Job drawing, mm, ordinate dimensions from the low corner. One solid piece. Give positions to 0.01 mm unless a question says otherwise; leave off trailing zeros. Order: outer loops, then holes, each group sorted by start corner. A loop starts at its lowest first (then second) coordinate and runs counter-clockwise, first axis right, second up. Notation, with made-up numbers: (6.5, 26.25) - (47.5, 26.25) arc R9 cw to (47.5, 31.25) - close; hole circle Ø10 at (70.5, 16.25). An arc over 180 degrees is marked (long way). Use a Markdown table: item, result. Add a question column.
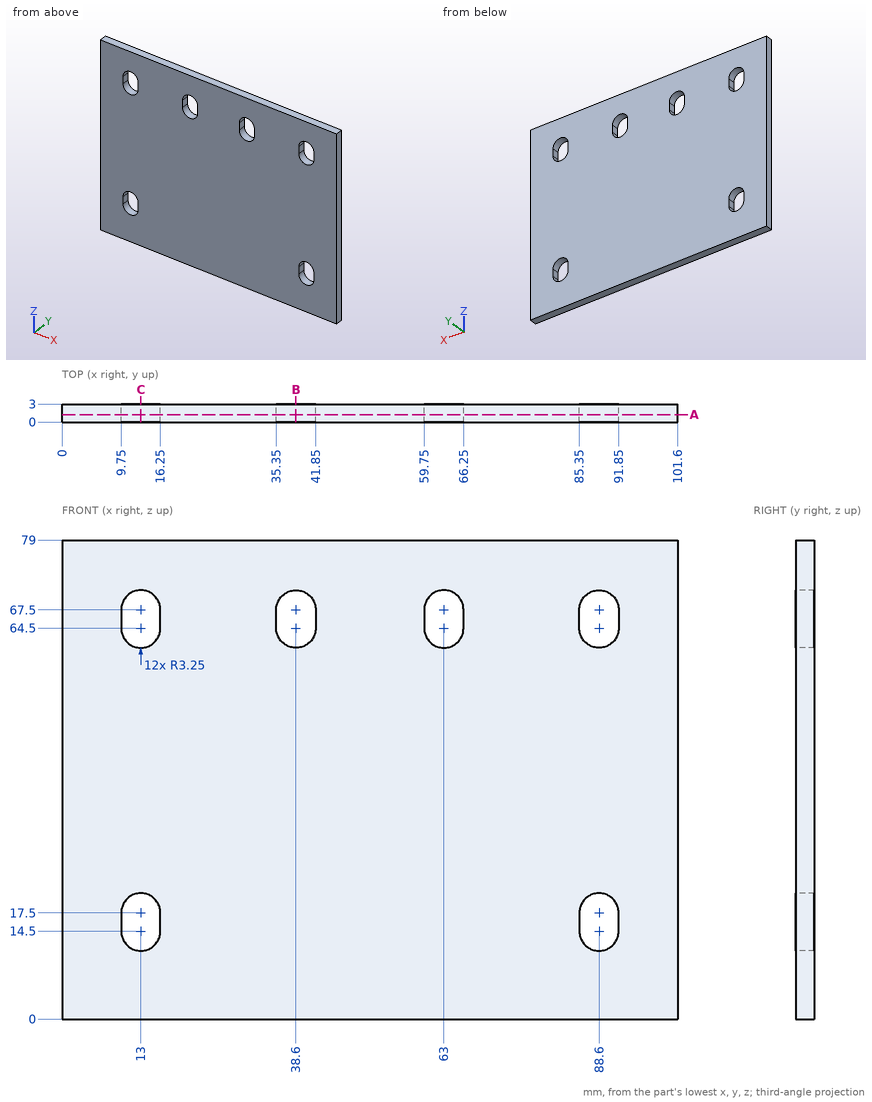
1. Cut at B-B (x = 38.6). Write the cut outline in (y, z), plus the area to 4 significant figures.
2. Cut at A-A (y = 1.25). Write the cut outline in (x, z).
3. Drill centre lines: probe 1 along X at (y, z) = (2.15, 19); probe 2 along X at (y, z) = (0.95, 19.5); probe 3 along X at (y, z) = (0.2, 62.5). Where is each one in solid material? Low to high. Write a range as [from, to].
4. Cut at C-C (x = 13). Write the cut outline in (y, z).
Responses:
| question | item | result |
|---|---|---|
| 1 | outline | (0, 0) - (3, 0) - (3, 61.25) - (0, 61.25) - close; (0, 70.75) - (3, 70.75) - (3, 79) - (0, 79) - close |
| 1 | area | 208.5 mm² |
| 2 | outline | (0, 0) - (101.6, 0) - (101.6, 79) - (0, 79) - close; hole (9.75, 14.5) arc R3.25 ccw to (16.25, 14.5) - (16.25, 17.5) arc R3.25 ccw to (9.75, 17.5) - close; hole (9.75, 64.5) arc R3.25 ccw to (16.25, 64.5) - (16.25, 67.5) arc R3.25 ccw to (9.75, 67.5) - close; hole (35.35, 64.5) arc R3.25 ccw to (41.85, 64.5) - (41.85, 67.5) arc R3.25 ccw to (35.35, 67.5) - close; hole (59.75, 64.5) arc R3.25 ccw to (66.25, 64.5) - (66.25, 67.5) arc R3.25 ccw to (59.75, 67.5) - close; hole (85.35, 14.5) arc R3.25 ccw to (91.85, 14.5) - (91.85, 17.5) arc R3.25 ccw to (85.35, 17.5) - close; hole (85.35, 64.5) arc R3.25 ccw to (91.85, 64.5) - (91.85, 67.5) arc R3.25 ccw to (85.35, 67.5) - close |
| 3 | probe 1 | x = [0, 10.12], [15.88, 85.72], [91.48, 101.6] |
| 3 | probe 2 | x = [0, 10.44], [15.56, 86.04], [91.16, 101.6] |
| 3 | probe 3 | x = [0, 10.44], [15.56, 36.04], [41.16, 60.44], [65.56, 86.04], [91.16, 101.6] |
| 4 | outline | (0, 0) - (3, 0) - (3, 11.25) - (0, 11.25) - close; (0, 20.75) - (3, 20.75) - (3, 61.25) - (0, 61.25) - close; (0, 70.75) - (3, 70.75) - (3, 79) - (0, 79) - close |
